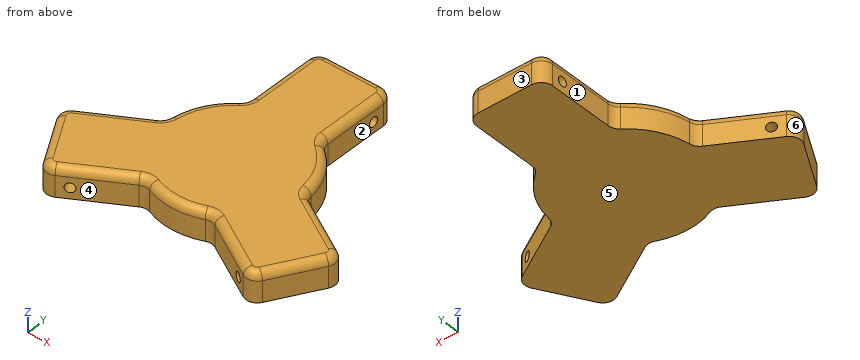
```python
from build123d import *

# Parameters (mm, degrees)
BOSS_EXTRUDE1_DEPTH = 9.525
FILLET1_R           = 2.54
SKETCH3_R           = 1.55
CUT_EXTRUDE2_DEPTH  = 5.08
CUT_EXTRUDE3_START  = -5.08
SKETCH4_R           = 1.55
CUT_EXTRUDE3_DEPTH  = 5.08
CIRPATTERN2_COUNT   = 3


with BuildPart() as part:
    # Sketch1 → Boss-Extrude1 (new body)
    with BuildSketch(Plane.XY):
        with BuildLine():
            Line((12.7, 21.969079793), (12.7, 43.5864))
            ThreePointArc((12.7, 43.5864), (11.584076836, 46.280476836), (8.89, 47.3964))
            Line((8.89, 47.3964), (-8.89, 47.3964))
            ThreePointArc((-8.89, 47.3964), (-11.584076836, 46.280476836), (-12.7, 43.5864))
            Line((-12.7, 43.5864), (-12.7, 21.969079793))
            ThreePointArc((-12.7, 21.969079793), (-13.101409662, 20.266842468), (-14.221056121, 18.923289925))
            ThreePointArc((-14.221056121, 18.923289925), (-20.499926929, 11.835638331), (-23.498577859, 2.854150907))
            ThreePointArc((-23.498577859, 2.854150907), (-24.102305263, 1.212732359), (-25.375781199, 0.013982731))
            Line((-25.375781199, 0.013982731), (-44.09692966, -10.794677372))
            ThreePointArc((-44.09692966, -10.794677372), (-45.872107058, -13.108133599), (-45.491486448, -15.99923416))
            Line((-45.491486448, -15.99923416), (-36.601486448, -31.39716584))
            ThreePointArc((-36.601486448, -31.39716584), (-34.288030221, -33.172343238), (-31.39692966, -32.791722628))
            Line((-31.39692966, -32.791722628), (-12.675781199, -21.983062525))
            ThreePointArc((-12.675781199, -21.983062525), (-11.000895601, -21.479574827), (-9.277521738, -21.777440832))
            ThreePointArc((-9.277521738, -21.777440832), (0, -23.671276662), (9.277521738, -21.777440832))
            ThreePointArc((9.277521738, -21.777440832), (11.000895601, -21.479574827), (12.675781199, -21.983062525))
            Line((12.675781199, -21.983062525), (31.39692966, -32.791722628))
            ThreePointArc((31.39692966, -32.791722628), (34.288030221, -33.172343238), (36.601486448, -31.39716584))
            Line((36.601486448, -31.39716584), (45.491486448, -15.99923416))
            ThreePointArc((45.491486448, -15.99923416), (45.872107058, -13.108133599), (44.09692966, -10.794677372))
            Line((44.09692966, -10.794677372), (25.375781199, 0.013982731))
            ThreePointArc((25.375781199, 0.013982731), (24.102305263, 1.212732359), (23.498577859, 2.854150907))
            ThreePointArc((23.498577859, 2.854150907), (20.499926929, 11.835638331), (14.221056121, 18.923289925))
            ThreePointArc((14.221056121, 18.923289925), (13.101409662, 20.266842468), (12.7, 21.969079793))
        make_face()
    extrude(amount=BOSS_EXTRUDE1_DEPTH)

    # Fillet1
    fillet1_edges = [part.edges().sort_by_distance(p)[0] for p in [
        (-24.102305263, 1.212732359, 9.525),
        (-34.736355429, -5.39034732, 9.525),
        (-45.872107058, -13.108133599, 9.525),
        (-41.046486448, -23.6982, 9.525),
        (-34.288030221, -33.172343238, 9.525),
        (-22.036355429, -27.387392576, 9.525),
        (-11.000895601, -21.479574827, 9.525),
        (0, -23.671276662, 9.525),
        (11.000895601, -21.479574827, 9.525),
        (22.036355429, -27.387392576, 9.525),
        (-13.101409662, 20.266842468, 9.525),
        (34.288030221, -33.172343238, 9.525),
        (41.046486448, -23.6982, 9.525),
        (45.872107058, -13.108133599, 9.525),
        (34.736355429, -5.39034732, 9.525),
        (24.102305263, 1.212732359, 9.525),
        (20.499926929, 11.835638331, 9.525),
        (13.101409662, 20.266842468, 9.525),
        (12.7, 32.777739897, 9.525),
        (11.584076836, 46.280476836, 9.525),
        (0, 47.3964, 9.525),
        (-20.499926929, 11.835638331, 9.525),
        (-11.584076836, 46.280476836, 9.525),
        (-12.7, 32.777739897, 9.525),
    ]]
    fillet(fillet1_edges, radius=FILLET1_R)

    # Sketch3 → Cut-Extrude2 (cut)
    with BuildSketch(Plane(origin=(-6.35, -10.998522628, 0), x_dir=(0.8660254037844575, -0.4999999999999674, 0), z_dir=(-0.4999999999999675, -0.8660254037844576, 0))):
        with Locations((39.7764, 3.582)):
            Circle(SKETCH3_R)
    cut_extrude2 = extrude(amount=-CUT_EXTRUDE2_DEPTH, mode=Mode.SUBTRACT)

    # Sketch4 → Cut-Extrude3 (cut)
    with BuildSketch(Plane(origin=(6.35, 10.998522628, 0), x_dir=(0.8660254037844387, -0.49999999999999983, 0), z_dir=(0.49999999999999983, 0.8660254037844387, 0)).offset(CUT_EXTRUDE3_START)):
        with Locations((39.7764, -3.582)):
            Circle(SKETCH4_R)
    cut_extrude3 = extrude(amount=CUT_EXTRUDE3_DEPTH, mode=Mode.SUBTRACT)

    # CirPattern2: Cut-Extrude2, Cut-Extrude3 ×3 about axis
    cirpattern2_axis = Axis((0, 0, 0), (0, 0, 1))
    add([cut_extrude2.rotate(cirpattern2_axis, i * 360 / CIRPATTERN2_COUNT) for i in range(1, CIRPATTERN2_COUNT)], mode=Mode.SUBTRACT)
    add([cut_extrude3.rotate(cirpattern2_axis, i * 360 / CIRPATTERN2_COUNT) for i in range(1, CIRPATTERN2_COUNT)], mode=Mode.SUBTRACT)


solid = part.part
```
Read the model definition and answer for the solid it produces. Units are mm, in the model's axes. Face numbers are marked on the shaded views. A direction names the side the tool comes from. Round coordinates to 2 decimals unless told otherwise and drop trailing zeros. Write each loop counter-clockwise with the first axis right and the second up, starting at its lowest first coordinate (ties: lowest second). Pieces come first, ordered by that corner, then holes. Notation, with made-up numbers: (51.25, 29) -> (57.25, 29) arc R24 ccw to (57.25, 62) -> close; hole circle Ø10 at (72, -11). An arc over 180 degrees is marked (long way). Answer in a Markdown table with one row per item. Add a question column.
1) Determine the mould class of the marked faces 4, 5 and 6 for opening direction X: pulls with the +X half, pulls with the -X half, needs draft (parallel to the pull), parting line crosses it, or undercut.
2) Given P1, Ø3.5, axis at y = 30, z = 3.5, coming from the -X side; P2, Ø5, axis at y = 17.5, z = 6.5, coming from the +X side; P3, Ø1.9, axis at y = 39.78, z = 3.58, coming from the -X side, each flat-ended and moving along its own axis, determine where each tip first touches the part or whether it passes through.
3) Find section A-A, the plane z = 1. Determine the outline of the cut face in (x, y).
4) Find section B-B, the plane y = 27. Determine the outline of the cut face in (x, z) (3 decimals).
5) Which of the six approach directions +Z, -Z, +X, -X, +Y, -Y give full straight-line access (tool end or side, diameter ignored) to the marked faces 1, 2 and 3?
6) Consider line 1 (X direction, y = 0, z = 2); line 2 (Y direction, x = 3, z = 3.25); line 3 (X direction, y = 3.5, z = 3). Determine where each line is inside the solid, lowest interval first.
7) Find section C-C, the plane x = 0. Determine the outline of the cut face in (y, z) (3 decimals), and give its area (3 significant figures).
Findings below:
| question | item | result |
|---|---|---|
| 1 | face 4 | undercut |
| 1 | face 5 | needs draft |
| 1 | face 6 | pulls with the -X half |
| 2 | P1 | x = -12.7 |
| 2 | P2 | x = 18.31 |
| 2 | P3 | x = -7.62 |
| 3 | outline | (-45.49, -16) -> (-36.6, -31.4) arc R3.81 ccw to (-31.4, -32.79) -> (-12.68, -21.98) arc R3.81 cw to (-9.28, -21.78) arc R23.67 ccw to (9.28, -21.78) arc R3.81 cw to (12.68, -21.98) -> (31.4, -32.79) arc R3.81 ccw to (36.6, -31.4) -> (45.49, -16) arc R3.81 ccw to (44.1, -10.79) -> (25.38, 0.01) arc R3.81 cw to (23.5, 2.85) arc R23.67 ccw to (14.22, 18.92) arc R3.81 cw to (12.7, 21.97) -> (12.7, 43.59) arc R3.81 ccw to (8.89, 47.4) -> (-8.89, 47.4) arc R3.81 ccw to (-12.7, 43.59) -> (-12.7, 21.97) arc R3.81 cw to (-14.22, 18.92) arc R23.67 ccw to (-23.5, 2.85) arc R3.81 cw to (-25.38, 0.01) -> (-44.1, -10.79) arc R3.81 ccw to start |
| 4 | outline | (-12.7, 0) -> (12.7, 0) -> (12.7, 6.985) arc R2.54 ccw to (10.16, 9.525) -> (-10.16, 9.525) arc R2.54 ccw to (-12.7, 6.985) -> close |
| 5 | face 1 | +Z, -Z, -X, +Y |
| 5 | face 2 | +Z, -Z, +X, +Y |
| 5 | face 3 | +Z, -Z, +X, -X, +Y |
| 6 | line 1 | -25.4 to 25.4 |
| 6 | line 2 | -23.48 to 47.4 |
| 6 | line 3 | -23.41 to 23.41 |
| 7 | outline | (-23.671, 0) -> (47.396, 0) -> (47.396, 6.985) arc R2.54 ccw to (44.856, 9.525) -> (-21.131, 9.525) arc R2.54 ccw to (-23.671, 6.985) -> close |
| 7 | area | 674 mm² |
